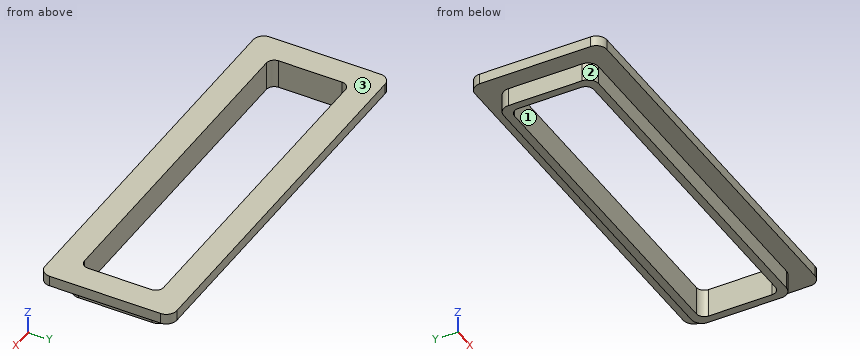
```python
from build123d import *

# Parameters (mm, degrees)
F0_W     = 75
F0_H     = 25
F0_W_2   = 65
F0_H_2   = 15
F1_DEPTH = 2
F2_R     = 2
F3_W     = 68
F3_H     = 18
F3_W_2   = 65
F3_H_2   = 15
F4_DEPTH = 3.5
F5_R     = 2
F6_R     = 1.5


with BuildPart() as f1:
    # F0 (on Top) → F1 (new body)
    with BuildSketch(Plane.XY):
        Rectangle(F0_W, F0_H)
        Rectangle(F0_W_2, F0_H_2, mode=Mode.SUBTRACT)
    extrude(amount=F1_DEPTH)

    # F2
    f2_edges = [f1.edges().sort_by_distance(p)[0] for p in [
        (37.5, 12.5, 1),
        (37.5, -12.5, 1),
        (-37.5, -12.5, 1),
        (-37.5, 12.5, 1),
    ]]
    fillet(f2_edges, radius=F2_R)

    # F3 (on face) → F4 (join)
    with BuildSketch(Plane(origin=(0, 0, 0), x_dir=(1, 0, 0), z_dir=(0, 0, -1))):
        Rectangle(F3_W, F3_H)
        Rectangle(F3_W_2, F3_H_2, mode=Mode.SUBTRACT)
    extrude(amount=F4_DEPTH)

    # F5
    f5_edges = [f1.edges().sort_by_distance(p)[0] for p in [
        (34, -9, -1.75),
        (-34, -9, -1.75),
        (-34, 9, -1.75),
        (34, 9, -1.75),
    ]]
    fillet(f5_edges, radius=F5_R)

    # F6
    f6_edges = [f1.edges().sort_by_distance(p)[0] for p in [
        (32.5, 7.5, -0.75),
        (32.5, -7.5, -0.75),
        (-32.5, -7.5, -0.75),
        (-32.5, 7.5, -0.75),
    ]]
    fillet(f6_edges, radius=F6_R)


solid = f1.part
```
The listing builds one solid part. Answer for the finished solid, in the listing's coordinates (mm). Face numbers are marked on the shaded views. A direction names the side the tool comes from. Give positions to 0.01 mm unless a question says otherwise; leave off trailing zeros. Order: outer loops, then holes, each group sorted by start corner. A loop starts at its lowest first (then second) coordinate and runs counter-clockwise, first axis right, second up. Notation, with made-up numbers: (21.5, 45.5) -> (59.5, 45.5) arc R11 ccw to (59.5, 56.5) -> close; hole circle Ø1 at (-17, 64.25). An arc over 180 degrees is marked (long way). Answer as a JSON object with one key per item and string values. Group by question number.
Item 1: The part is cut by section C-C on z = 1.05. Write down the section's boundary in (x, y), and give its area (4 significant figures).
Item 2: The part is cut by section D-D on z = -2.25. Write down the section's boundary in (x, y), and give its area (3 significant figures).
Item 3: The part is cut by section B-B on x = 13. Write down the section's boundary in (y, z).
Item 4: The part is cut by section A-A on y = -3.75. Write down the section's boundary in (x, z), and give its area (3 significant figures).
Item 5: A tool of negligible diameter and unlimited length cuts with its end or side. For the marked faces 1, 2 and 3, from which of +Z, -Z, +X, -X, +Y, -Y can it reach the whole face along a straight path? Write none if from no direction.
Item 6: Flat-ended cylindrical pins translate along their axes: pin 1 (1.5 mm diameter, centred on y = -3, z = -1, fed in from +X); pin 2 (1.8 mm diameter, centred on x = 0.5, z = -1, fed in from +Y); pin 3 (2 mm diameter, centred on x = -4, z = -3, fed in from -Y). Find the tip coordinate at first contact, or state that the pin passes through.
Item 7: Consider L1, parallel to Y at x = 18, z = -2.1; L2, parallel to X at y = -2, z = -0.55; L3, parallel to X at y = -4, z = 1.2. Determine where each line is inside the solid, lowest interval first. Write a range as from..to.
Result set:
{
 "1": {"outline": "(-37.5, -10.5) arc R2 ccw to (-35.5, -12.5) -> (35.5, -12.5) arc R2 ccw to (37.5, -10.5) -> (37.5, 10.5) arc R2 ccw to (35.5, 12.5) -> (-35.5, 12.5) arc R2 ccw to (-37.5, 10.5) -> close; hole (-32.5, -6) arc R1.5 ccw to (-31, -7.5) -> (31, -7.5) arc R1.5 ccw to (32.5, -6) -> (32.5, 6) arc R1.5 ccw to (31, 7.5) -> (-31, 7.5) arc R1.5 ccw to (-32.5, 6) -> close", "area": "898.5 mm²"},
 "2": {"outline": "(-34, -7) arc R2 ccw to (-32, -9) -> (32, -9) arc R2 ccw to (34, -7) -> (34, 7) arc R2 ccw to (32, 9) -> (-32, 9) arc R2 ccw to (-34, 7) -> close; hole (-32.5, -6) arc R1.5 ccw to (-31, -7.5) -> (31, -7.5) arc R1.5 ccw to (32.5, -6) -> (32.5, 6) arc R1.5 ccw to (31, 7.5) -> (-31, 7.5) arc R1.5 ccw to (-32.5, 6) -> close", "area": "247 mm²"},
 "3": {"outline": "(-12.5, 0) -> (-9, 0) -> (-9, -3.5) -> (-7.5, -3.5) -> (-7.5, 2) -> (-12.5, 2) -> close; (7.5, -3.5) -> (9, -3.5) -> (9, 0) -> (12.5, 0) -> (12.5, 2) -> (7.5, 2) -> close"},
 "4": {"outline": "(-37.5, 0) -> (-34, 0) -> (-34, -3.5) -> (-32.5, -3.5) -> (-32.5, 2) -> (-37.5, 2) -> close; (32.5, -3.5) -> (34, -3.5) -> (34, 0) -> (37.5, 0) -> (37.5, 2) -> (32.5, 2) -> close", "area": "30.5 mm²"},
 "5": {"face 1": "+Z, -Z", "face 2": "-Z, -X, -Y", "face 3": "+Z, +X, -X, +Y, -Y"},
 "6": {"pin 1": "x = 34", "pin 2": "y = 9", "pin 3": "y = -9"},
 "7": {"L1": "-9..-7.5, 7.5..9", "L2": "-34..-32.5, 32.5..34", "L3": "-37.5..-32.5, 32.5..37.5"}
}
